from build123d import *

# Parameters (mm, degrees)
SKETCH1_W            = 50.8
SKETCH1_H            = 50.8
SKETCH1_W_2          = 44.45
SKETCH1_H_2          = 44.45
BOSS_EXTRUDE1_DEPTH  = 304.8
SKETCH2_R            = 3.175
CUT_EXTRUDE1_DEPTH   = 101.6
LPATTERN1_COUNT      = 3
LPATTERN1_PITCH      = 19.05
LPATTERN1_COUNT_DIR2 = 2
LPATTERN1_PITCH_DIR2 = 19.05
CUT_EXTRUDE2_DEPTH   = 311.04651264
SKETCH4_R            = 2.5527
CUT_EXTRUDE3_DEPTH   = 50.8
LPATTERN2_COUNT      = 3
LPATTERN2_PITCH      = 25.4
LPATTERN2_COUNT_DIR2 = 2
LPATTERN2_PITCH_DIR2 = 25.4


with BuildPart() as part:
    # Sketch1 → Boss-Extrude1 (new body)
    with BuildSketch(Plane(origin=(0, 0, 0), x_dir=(1, 0, 0), z_dir=(0, 1, 0))):
        Rectangle(SKETCH1_W, SKETCH1_H)
        Rectangle(SKETCH1_W_2, SKETCH1_H_2, mode=Mode.SUBTRACT)
    extrude(amount=BOSS_EXTRUDE1_DEPTH)

    # Sketch2 → Cut-Extrude1 (cut)
    with BuildSketch(Plane.XY.offset(25.4)):
        with Locations((-19.05, 292.1)):
            Circle(SKETCH2_R)
    cut_extrude1 = extrude(amount=-CUT_EXTRUDE1_DEPTH, mode=Mode.SUBTRACT)

    # LPattern1: Cut-Extrude1 3 × 2
    with Locations(*[(i * LPATTERN1_PITCH, -j * LPATTERN1_PITCH_DIR2, 0) for i in range(LPATTERN1_COUNT) for j in range(LPATTERN1_COUNT_DIR2) if (i, j) != (0, 0)]):
        add(cut_extrude1, mode=Mode.SUBTRACT)

    # Sketch3 → Cut-Extrude2 (cut, through all)
    with BuildSketch(Plane(origin=(25.4, 0, 0), x_dir=(0, 0, -1), z_dir=(1, 0, 0))):
        Polygon((-3.666174209, 19.05), (3.666174209, 19.05), (7.332348419, 25.4), (3.666174209, 31.75), (-3.666174209, 31.75), (-7.332348419, 25.4), align=None)
    extrude(amount=-CUT_EXTRUDE2_DEPTH, mode=Mode.SUBTRACT)

    # Sketch4 → Cut-Extrude3 (cut)
    with BuildSketch(Plane(origin=(25.4, 0, 0), x_dir=(0, 0, -1), z_dir=(1, 0, 0))):
        with Locations((-12.7, 177.8)):
            Circle(SKETCH4_R)
    cut_extrude3 = extrude(amount=-CUT_EXTRUDE3_DEPTH, mode=Mode.SUBTRACT)

    # LPattern2: Cut-Extrude3 3 × 2
    with Locations(*[(0, -i * LPATTERN2_PITCH, -j * LPATTERN2_PITCH_DIR2) for i in range(LPATTERN2_COUNT) for j in range(LPATTERN2_COUNT_DIR2) if (i, j) != (0, 0)]):
        add(cut_extrude3, mode=Mode.SUBTRACT)


solid = part.part
CAD build for the part. Positions are in the model's coordinates, mm. Give positions to 0.01 mm unless a question says otherwise; leave off trailing zeros. Loops run counter-clockwise (first coordinate to the right, second up) from the corner with the lowest first, then second, coordinate; pieces in that order, holes last. Notation, with made-up numbers: M -25.75,-36.5 L 30.25,-36.5 A23 cw 30.25,-20.5 Z; hole C 58.25,81 d4. An arc over 180 degrees is marked long. One line per question, with ' | ' between items. Start each with the question number.
1. Saw through at B-B on z = 12.7. State how many separate pieces and enclosed holes the cut face has, plus the area to 3 significant figures.
2. Flat gauge pin, fed straight in: pin 1 (6.5 mm diameter, centred on y = 127, z = -12.7, fed in from +X). Where does the tip first touch, or does it go through?
3. Saw through at D-D on y = 230.5. Give the cut face in (x, z) (3 decimals), plus the area to 3 significant figures.
4. Saw through at A-A on x = -11. Give the cut face in (y, z) (3 decimals), plus the area to 3 significant figures.
5. Probe L1, parallel to X at y = 292.1, z = -23 (3 decimals); L2, parallel to Y at x = 0, z = -23 (3 decimals); L3, parallel to Y at x = 0.5, z = 22.5. List the from-to ranges inside material, lowest first. Write a range as from..to.
6. Saw through at C-C on y = 177.8. Give the cut face in (x, z) (3 decimals), plus the area to 3 significant figures.
7. Two-plate mould, pull along Y, no slides. Class faces 1 (the face through (0, 150, -22.225)), 2 (the face through (-23.79, 149.908, 13.253)), 3 (the face through (-23, 304.8, 0)): pulls with the +Y half, pulls with the -Y half, needs draft (parallel to the pull), parting line crosses it, or undercut.
Result sheet:
1) separate pieces: 8 | enclosed holes: 0 | area: 1,840 mm^2
2) pin 1: stops at x = 25.4
3) outline: M -25.4,-25.4 L 25.4,-25.4 L 25.4,25.4 L -25.4,25.4 Z; hole M -22.225,-22.225 L 22.225,-22.225 L 22.225,22.225 L -22.225,22.225 Z | area: 605 mm^2
4) outline: M 0,-25.4 L 304.8,-25.4 L 304.8,-22.225 L 0,-22.225 Z; M 0,22.225 L 304.8,22.225 L 304.8,25.4 L 0,25.4 Z | area: 1,940 mm^2
5) L1: x = -25.4..-22.225, -15.875..-3.175, 3.175..15.875, 22.225..25.4 | L2: y = 0..269.875, 276.225..288.925, 295.275..304.8 | L3: y = 0..269.91, 276.19..288.96, 295.24..304.8
6) outline: M -25.4,-25.4 L 25.4,-25.4 L 25.4,-15.253 L 22.225,-15.253 L 22.225,-22.225 L -22.225,-22.225 L -22.225,-15.253 L -25.4,-15.253 Z; M -25.4,-10.147 L -22.225,-10.147 L -22.225,10.147 L -25.4,10.147 Z; M -25.4,15.253 L -22.225,15.253 L -22.225,22.225 L 22.225,22.225 L 22.225,15.253 L 25.4,15.253 L 25.4,25.4 L -25.4,25.4 Z; M 22.225,-10.147 L 25.4,-10.147 L 25.4,10.147 L 22.225,10.147 Z | area: 540 mm^2
7) face 1: needs draft | face 2: undercut | face 3: pulls with the +Y half
